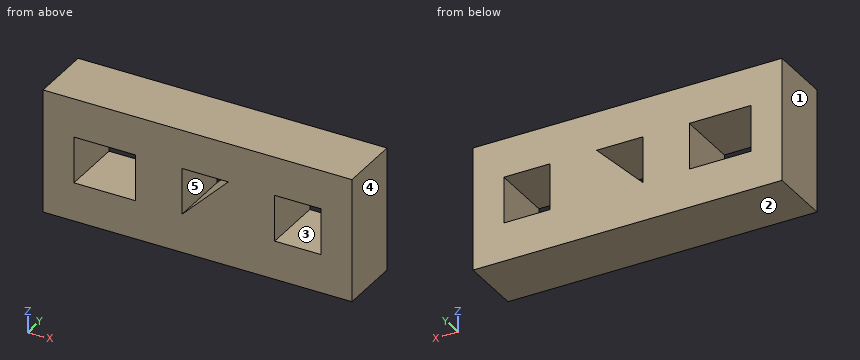
from build123d import *

# Parameters (mm, degrees)
SKETCH1_W           = 127
SKETCH1_H           = 50.8
BOSS_EXTRUDE1_DEPTH = 25.4
SKETCH2_W           = 25.4
SKETCH2_H           = 19.05
SKETCH2_W_2         = 19.05
CUT_EXTRUDE1_DEPTH  = 26.4


with BuildPart() as part:
    # Sketch1 → Boss-Extrude1 (new body)
    with BuildSketch(Plane(origin=(0, 0, 0), x_dir=(1, 0, 0), z_dir=(0, 1, 0))):
        with Locations((63.5, 25.4)):
            Rectangle(SKETCH1_W, SKETCH1_H)
    extrude(amount=BOSS_EXTRUDE1_DEPTH)

    # Sketch2 → Cut-Extrude1 (cut, through all)
    with BuildSketch(Plane(origin=(0, 25.4, 0), x_dir=(1, 0, 0), z_dir=(0, 1, 0))):
        Polygon((57.15, 34.925), (57.15, 15.875), (76.2, 15.875), align=None)
        with Locations((25.4, 25.4)):
            Rectangle(SKETCH2_W, SKETCH2_H)
        with Locations((104.775, 25.4)):
            Rectangle(SKETCH2_W_2, SKETCH2_H)
    extrude(amount=-CUT_EXTRUDE1_DEPTH, mode=Mode.SUBTRACT)


solid = part.part
Read the model definition and answer for the solid it produces. Units are mm, in the model's axes. Face numbers are marked on the shaded views. A direction names the side the tool comes from. Coordinates: 2 decimals unless noted, no trailing zeros. Order: outer loops, then holes, each group sorted by start corner. A loop starts at its lowest first (then second) coordinate and runs counter-clockwise, first axis right, second up. Notation, with made-up numbers: (89.5, -16) -> (108.5, -16) arc R31 ccw to (108.5, 12) -> close; hole circle Ø10 at (19.5, 74). An arc over 180 degrees is marked (long way). Answer as a JSON object with one key per item and string values.
1) A cutting plane is placed at C-C, the plane z = -25. Determine the outline of the cut face in (x, y) (3 decimals).
Model answer:
{"outline": "(0, 0) -> (12.7, 0) -> (12.7, 25.4) -> (0, 25.4) -> close; (38.1, 0) -> (57.15, 0) -> (57.15, 25.4) -> (38.1, 25.4) -> close; (67.075, 0) -> (95.25, 0) -> (95.25, 25.4) -> (67.075, 25.4) -> close; (114.3, 0) -> (127, 0) -> (127, 25.4) -> (114.3, 25.4) -> close"}
2) A tool of negligible diameter and unlimited length cuts with its end or side. For the marked faces 4 and 5, from which of +Z, -Z, +X, -X, +Y, -Y can it reach the whole face along a straight path? Write none if from no direction.
Model answer:
{"face 4": "+Z, -Z, +X, +Y, -Y", "face 5": "+Y, -Y"}
3) Consider line 1 along Z through (x, y) = (20.5, 1.5) (3 decimals); line 2 along X through (y, z) = (16, -24) (3 decimals); line 3 along Z through (x, y) = (59.5, 1.5) (3 decimals). Determine where each line is inside the solid, lowest interval first. Write a range as from..to.
Model answer:
{"line 1": "z = -50.8..-34.925, -15.875..0", "line 2": "x = 0..12.7, 38.1..57.15, 68.075..95.25, 114.3..127", "line 3": "z = -50.8..-32.575, -15.875..0"}
4) The mould has two halves that part along X. Classify the marked faces 1, 2 and 3: released by +X, released by -X, zero draft, split by the parting line, or undercut.
Model answer:
{"face 1": "released by -X", "face 2": "zero draft", "face 3": "undercut"}
5) A cutting plane is placed at A-A, the plane x = 31. Determine the outline of the cut face in (y, z) (3 decimals).
Model answer:
{"outline": "(0, -50.8) -> (25.4, -50.8) -> (25.4, -34.925) -> (0, -34.925) -> close; (0, -15.875) -> (25.4, -15.875) -> (25.4, 0) -> (0, 0) -> close"}
6) A cutting plane is placed at D-D, the plane x = 60. Determine the outline of the cut face in (y, z) (3 decimals).
Model answer:
{"outline": "(0, -50.8) -> (25.4, -50.8) -> (25.4, -32.075) -> (0, -32.075) -> close; (0, -15.875) -> (25.4, -15.875) -> (25.4, 0) -> (0, 0) -> close"}
7) A cutting plane is placed at B-B, the plane y = 3.5. Determine the outline of the cut face in (x, z) (3 decimals).
Model answer:
{"outline": "(0, -50.8) -> (127, -50.8) -> (127, 0) -> (0, 0) -> close; hole (12.7, -34.925) -> (38.1, -34.925) -> (38.1, -15.875) -> (12.7, -15.875) -> close; hole (57.15, -34.925) -> (76.2, -15.875) -> (57.15, -15.875) -> close; hole (95.25, -34.925) -> (114.3, -34.925) -> (114.3, -15.875) -> (95.25, -15.875) -> close"}
